```python
from build123d import *

# Parameters (mm, degrees)
SKETCH1_W           = 90
SKETCH1_H           = 10
BOSS_EXTRUDE1_DEPTH = 22.8
SKETCH2_R           = 1.5
CUT_EXTRUDE1_DEPTH  = 23.8
LPATTERN1_COUNT     = 9
LPATTERN1_PITCH     = 10
SKETCH3_W           = 10
SKETCH3_H           = 10
CUT_EXTRUDE2_DEPTH  = 91
SKETCH4_W           = 90
SKETCH4_H           = 22.8
BOSS_EXTRUDE2_DEPTH = 10


with BuildPart() as part:
    # Sketch1 → Boss-Extrude1 (new body)
    with BuildSketch(Plane(origin=(0, 0, 0), x_dir=(1, 0, 0), z_dir=(0, 1, 0))):
        Rectangle(SKETCH1_W, SKETCH1_H)
    extrude(amount=BOSS_EXTRUDE1_DEPTH)

    # Sketch2 → Cut-Extrude1 (cut, through all)
    with BuildSketch(Plane(origin=(0, 22.8, 0), x_dir=(1, 0, 0), z_dir=(0, 1, 0))):
        with Locations((-40, 0)):
            Circle(SKETCH2_R)
    cut_extrude1 = extrude(amount=-CUT_EXTRUDE1_DEPTH, mode=Mode.SUBTRACT)

    # LPattern1: Cut-Extrude1 ×9
    with Locations(*[(i * LPATTERN1_PITCH, 0, 0) for i in range(1, LPATTERN1_COUNT)]):
        add(cut_extrude1, mode=Mode.SUBTRACT)

    # Sketch3 → Cut-Extrude2 (cut, through all)
    with BuildSketch(Plane(origin=(45, 0, 0), x_dir=(0, 0, -1), z_dir=(1, 0, 0))):
        with Locations((0, 11.4)):
            Rectangle(SKETCH3_W, SKETCH3_H)
    extrude(amount=-CUT_EXTRUDE2_DEPTH, mode=Mode.SUBTRACT)

    # Sketch4 → Boss-Extrude2 (add)
    with BuildSketch(Plane.XY.offset(5)):
        with Locations((0, 11.4)):
            Rectangle(SKETCH4_W, SKETCH4_H)
    extrude(amount=BOSS_EXTRUDE2_DEPTH)


solid = part.part
```
The listing builds one solid part. Answer for the finished solid, in the listing's coordinates (mm). Coordinates: 2 decimals unless noted, no trailing zeros. Loops run counter-clockwise (first coordinate to the right, second up) from the corner with the lowest first, then second, coordinate; pieces in that order, holes last. Notation, with made-up numbers: (44.5, 67.25) -> (101.5, 67.25) arc R24 cw to (101.5, 81.25) -> close; hole circle Ø2 at (9, 50.25). An arc over 180 degrees is marked (long way). Return JSON: item names as keys, results as strings. Group by question number.
(1) A cutting plane is placed at B-B on y = 20. Count the separate pieces of the cut face and the enclosed holes in it, and give its area (3 significant figures).
(2) Determine the mould class of faces 1 (the flat face through (-1, 11, 5)), 2 (the cylindrical face through (-11.2, 3.2, 0.9)), 3 (the cylindrical face through (-31.2, 3.2, 0.9)), 4 (the flat face through (1, 16.4, 2)) for opening direction Z: released by +Z, released by -Z, zero draft, split by the parting line, or undercut.
(3) A cutting plane is placed at C-C on x = 40. Write down the section's boundary in (y, z).
(4) A cutting plane is placed at D-D on x = -33. Write down the section's boundary in (y, z), and give its area (3 significant figures).
(5) Find the intervals of material crossed by probe 1 along Z at (x, y) = (-30, 19); probe 2 along Y at (x, z) = (1.5, 3.25); probe 3 along Z at (x, y) = (21, 1.5), in increasing order. Write a range as from..to.
(6) A cutting plane is placed at A-A on z = -2.5. Write down the section's boundary in (x, y).
The answers:
{
 "1": {"separate pieces": "1", "enclosed holes": "9", "area": "1,740 mm^2"},
 "2": {"face 1": "released by -Z", "face 2": "undercut", "face 3": "undercut", "face 4": "zero draft"},
 "3": {"outline": "(0, -5) -> (6.4, -5) -> (6.4, -1.5) -> (0, -1.5) -> close; (0, 1.5) -> (6.4, 1.5) -> (6.4, 5) -> (16.4, 5) -> (16.4, 1.5) -> (22.8, 1.5) -> (22.8, 15) -> (0, 15) -> close; (16.4, -5) -> (22.8, -5) -> (22.8, -1.5) -> (16.4, -1.5) -> close"},
 "4": {"outline": "(0, -5) -> (6.4, -5) -> (6.4, 5) -> (16.4, 5) -> (16.4, -5) -> (22.8, -5) -> (22.8, 15) -> (0, 15) -> close", "area": "356 mm^2"},
 "5": {"probe 1": "z = -5..-1.5, 1.5..15", "probe 2": "y = 0..6.4, 16.4..22.8", "probe 3": "z = -5..-1.12, 1.12..15"},
 "6": {"outline": "(-45, 0) -> (45, 0) -> (45, 6.4) -> (-45, 6.4) -> close; (-45, 16.4) -> (45, 16.4) -> (45, 22.8) -> (-45, 22.8) -> close"}
}
